Build history of the part. All positions in model axes, mm. A direction names the side the tool comes from. Coordinates: 2 decimals unless noted, no trailing zeros. Return JSON: item names as keys, results as strings.
Autodesk Inventor part; units mm, degrees
ref_plane "YZ Plane" through (0, 0, 0) normal (1, 0, 0) x (0, 1, 0)
ref_plane "XZ Plane" through (0, 0, 0) normal (0, 1, 0) x (-1, 0, 0)
ref_plane "XY Plane" through (0, 0, 0) normal (0, 0, 1) x (1, 0, 0)
sketch "Skizze1" plane through (0, 0, 0) normal (0, 1, 0) x (-1, 0, 0)
  line L0 (387.1429, -272.5) -> (87.1429, -272.5)
  line L1 (87.1429, -272.5) -> (87.1429, -572.5)
  line L2 (87.1429, -572.5) -> (387.1429, -572.5)
  line L3 (387.1429, -572.5) -> (387.1429, -272.5)
  circle A0 centre (107.1429, -292.5) radius 3.75
  circle A1 centre (367.1429, -292.5) radius 3.75
  circle A2 centre (367.1429, -552.5) radius 3.75
  circle A3 centre (107.1429, -552.5) radius 3.75
  line L4 (387.1429, -297.5) -> (362.1429, -297.5)
  line L5 (362.1429, -297.5) -> (362.1429, -287.5)
  line L6 (362.1429, -287.5) -> (387.1429, -287.5)
  line L7 (387.1429, -287.5) -> (387.1429, -297.5)
  line L8 (362.1429, -272.5) -> (372.1429, -272.5)
  line L9 (372.1429, -272.5) -> (372.1429, -297.5)
  line L10 (372.1429, -297.5) -> (362.1429, -297.5)
  line L11 (362.1429, -297.5) -> (362.1429, -272.5)
  line L12 (362.1429, -572.5) -> (372.1429, -572.5)
  line L13 (372.1429, -572.5) -> (372.1429, -547.5)
  line L14 (372.1429, -547.5) -> (362.1429, -547.5)
  line L15 (362.1429, -547.5) -> (362.1429, -572.5)
  line L16 (387.1429, -547.5) -> (362.1429, -547.5)
  line L17 (362.1429, -547.5) -> (362.1429, -557.5)
  line L18 (362.1429, -557.5) -> (387.1429, -557.5)
  line L19 (387.1429, -557.5) -> (387.1429, -547.5)
  line L20 (112.1429, -547.5) -> (87.1429, -547.5)
  line L21 (87.1429, -547.5) -> (87.1429, -557.5)
  line L22 (87.1429, -557.5) -> (112.1429, -557.5)
  line L23 (112.1429, -557.5) -> (112.1429, -547.5)
  line L24 (112.1429, -547.5) -> (102.1429, -547.5)
  line L25 (102.1429, -547.5) -> (102.1429, -572.5)
  line L26 (102.1429, -572.5) -> (112.1429, -572.5)
  line L27 (112.1429, -572.5) -> (112.1429, -547.5)
  line L28 (112.1429, -287.5) -> (87.1429, -287.5)
  line L29 (87.1429, -287.5) -> (87.1429, -297.5)
  line L30 (87.1429, -297.5) -> (112.1429, -297.5)
  line L31 (112.1429, -297.5) -> (112.1429, -287.5)
  line L32 (112.1429, -297.5) -> (102.1429, -297.5)
  line L33 (102.1429, -297.5) -> (102.1429, -272.5)
  line L34 (102.1429, -272.5) -> (112.1429, -272.5)
  line L35 (112.1429, -272.5) -> (112.1429, -297.5)
  circle A4 centre (367.1429, -552.5) radius 5
  circle A5 centre (107.1429, -552.5) radius 5
  circle A6 centre (107.1429, -292.5) radius 5
  circle A7 centre (367.1429, -292.5) radius 5
  point P0 (0, 0)
  dimension "d0" = 300
  dimension "d1" = 300
  dimension "d2" = 7.5
  dimension "d3" = 7.5
  dimension "d4" = 7.5
  dimension "d5" = 7.5
  dimension "d6" = 20
  dimension "d7" = 20
  dimension "d8" = 20
  dimension "d9" = 20
  dimension "d10" = 20
  dimension "d12" = 20
  dimension "d13" = 20
  dimension "d23" = 10
  dimension "d24" = 10
  dimension "d25" = 25
  dimension "d26" = 25
  dimension "d27" = 25
  dimension "d28" = 25
  dimension "d29" = 25
  dimension "d30" = 25
  dimension "d31" = 10
  dimension "d32" = 10
  dimension "d33" = 10
  dimension "d34" = 10
  dimension "d35" = 10
  dimension "d36" = 10
  dimension "d37" = 10
  dimension "d38" = 10
extrude "Extrusion1" add sketch "Skizze1" along normal blind 20 contours L3 L6 L9 L0 | L9 L6 L11 L0 | L3 L4 L9 L6 | L11 L5 L4 L3 L16 L14 L15 L2 L27 L23 L20 L1 L30 L31 L35 L0 | L9 A7 L6 | L35 L28 L33 L0 | L6 A7 L5 | A7 | L9 L4 A7 | L3 L18 L13 L16 | L33 L28 L1 L0 | L31 A6 L28 | A7 L4 L5 | L3 L2 L13 L18 | L13 A4 L14 | L33 L30 L1 L28 | L28 A6 L33 | A6 | L31 L30 A6 | L18 A4 L13 | L13 L2 L15 L18 | A4 | A4 L15 L14 | A6 L30 L33 | L18 L15 A4 | L20 L25 L22 L1 | L2 L25 L22 L27 | L22 L25 L2 L1 | L20 A5 L25 | L22 A5 L23 | L25 A5 L22 | L20 L23 A5 | A5 | A0 | A1 | A2 | A3
extrude "Extrusion2" cut sketch "Skizze1" along normal blind 3 contours L9 L6 L11 L0 | L3 L4 L9 L6 | L9 A7 L6 | L35 L28 L33 L0 | L6 A7 L5 | A7 | L9 L4 A7 | L3 L18 L13 L16 | L31 A6 L28 | A7 L4 L5 | L13 A4 L14 | L33 L30 L1 L28 | L28 A6 L33 | A6 | L31 L30 A6 | L18 A4 L13 | L13 L2 L15 L18 | A4 | A4 L15 L14 | A6 L30 L33 | L18 L15 A4 | L20 L25 L22 L1 | L2 L25 L22 L27 | L20 A5 L25 | L22 A5 L23 | L25 A5 L22 | L20 L23 A5 | A5 | A0 | A1 | A2 | A3
extrude "Extrusion3" cut sketch "Skizze1" along normal blind 10 contours A0 | A1 | A2 | A3
extrude "Extrusion4" cut sketch "Skizze1" along normal blind 6 contours A7 | A6 | A4 | A5
properties material "Holz (Kirsche)"
1. Mould opens along X. For faces 3 (the flat face through (-387.143, 10, -425)), 4 (the flat face through (-235, 20, -420)), 5 (the flat face through (-367, 10, -292)) say: pulls with the +X half, pulls with the -X half, needs draft (parallel to the pull), parting line crosses it, or undercut.
Check values:
{"face 3": "pulls with the -X half", "face 4": "needs draft", "face 5": "undercut"}
2. Probe L1, parallel to X at y = 8.9, z = -292.5; L2, parallel to X at y = 4, z = -292.5. List the from-to ranges inside material, lowest first.
Check values:
{"L1": "-387.14 to -370.89, -363.39 to -110.89, -103.39 to -87.14", "L2": "-387.14 to -372.14, -362.14 to -112.14, -102.14 to -87.14"}
3. Drop flat-ended pins along their axis: pin 1 (4.5 mm diameter, centred on x = -107.14, z = -552.5, fed in from -Y); pin 2 (7.5 mm diameter, centred on x = -369, z = -554, fed in from -Y). Give the stop position or say it passes through.
Check values:
{"pin 1": "y = 10", "pin 2": "y = 3"}
4. Tool access for faces 1 (the flat face through (-380, 0, -280)), 2 (the flat face through (-109, 6, -289)): list every direction of +Z, -Z, +X, -X, +Y, -Y with a clear straight run to the whole face (end or side of a thin tool).
Check values:
{"face 1": "+Z, -Z, +X, -X, -Y", "face 2": "-Y"}
